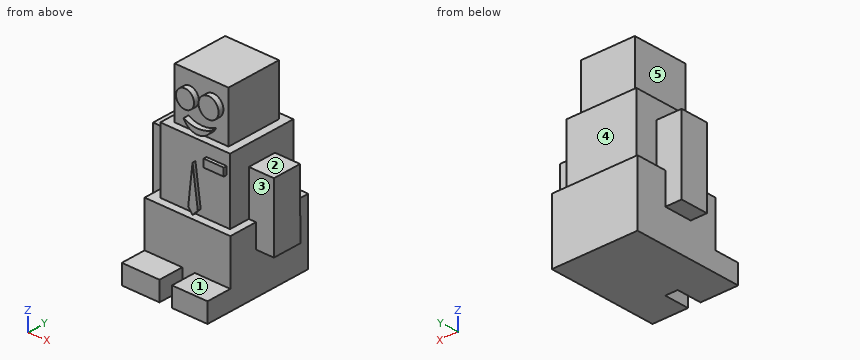
from build123d import *

# Parameters (mm, degrees)
F0_W      = 86.6950079799
F0_H      = 86.6950042546
F1_DEPTH  = 64.9986
F2_W      = 70.5124139786
F2_H      = 70.5124102533
F3_DEPTH  = 64.9986
F4_W      = 54.395288229
F4_H      = 56.1221279204
F5_DEPTH  = 50.8
F6_R      = 9.1186421801
F6_R_2    = 10.1513194638
F6_W      = 20.3841309994
F6_H      = 7.7653825283
F7_DEPTH  = 25.4
F8_W      = 29.1201900691
F8_H      = 44.812363273
F9_DEPTH  = 25.4
F10_W     = 29.5586548746
F10_H     = 23.6200721203
F11_DEPTH = 25.4
F12_W     = 28.1495144591
F12_H     = 46.7537163557
F12_H_2   = 31.3854509233
F13_DEPTH = 25.4
F15_DEPTH = 25.4
F16_W     = 38.1280947477
F16_H     = 19.5383913815
F16_W_2   = 35.9481638297
F17_DEPTH = 25.4
F19_DEPTH = 20
F18_W     = 20.3841309994
F18_H     = 7.7653825283
F20_DEPTH = 15


with BuildPart() as f1:
    # F0 (on Top) → F1 (new body)
    with BuildSketch(Plane.XY):
        with Locations((-0.8532218635, 5.3543392569)):
            Rectangle(F0_W, F0_H)
    extrude(amount=F1_DEPTH)

    # F2 (on face) → F3 (join)
    with BuildSketch(Plane.XY.offset(64.9986)):
        with Locations((0, 4.8926975578)):
            Rectangle(F2_W, F2_H)
    extrude(amount=F3_DEPTH)

    # F4 (on face) → F5 (join)
    with BuildSketch(Plane.XY.offset(129.9972)):
        with Locations((0, 4.8926975578)):
            Rectangle(F4_W, F4_H)
    extrude(amount=F5_DEPTH)

    # F6 (on face) → F7 (join)
    with BuildSketch(Plane.XZ.offset(23.1683664024)):
        with Locations((-11.8907419965, 158.3446115255)):
            Circle(F6_R)
        with Locations((11.8907429278, 159.8006188869)):
            Circle(F6_R_2)
        Polygon((5.5813710205, 70.9840506315), (0.2426664723, 110.2963015437), (0.2426664723, 65.1600137353), align=None)
        Polygon((0.2426664723, 65.1600137353), (0.2426664723, 110.2963015437), (-4.1253603995, 70.9840506315), align=None)
        with Locations((21.5974720195, 114.1789928079)):
            Rectangle(F6_W, F6_H)
    extrude(amount=F7_DEPTH)

    # F8 (on face) → F9 (join)
    with BuildSketch(Plane.YZ.offset(35.2562069893)):
        with Locations((5.0960322842, 87.4047816365)):
            Rectangle(F8_W, F8_H)
    extrude(amount=F9_DEPTH)

    # F10 (on face) → F11 (join)
    with BuildSketch(Plane.YZ.offset(35.2562069893)):
        with Locations((5.3152646869, 53.1885639399)):
            Rectangle(F10_W, F10_H)
    extrude(amount=F11_DEPTH)

    # F12 (on face) → F13 (join)
    with BuildSketch(Plane(origin=(-35.2562069893, 0, 0), x_dir=(0, -1, 0), z_dir=(-1, 0, 0))):
        with Locations((-3.6400225945, 88.3754581779)):
            Rectangle(F12_W, F12_H)
        with Locations((-3.6400225945, 49.3058745384)):
            Rectangle(F12_W, F12_H_2)
    extrude(amount=F13_DEPTH)

    # F14 (on face) → F15 (join)
    with BuildSketch(Plane.XZ.offset(23.1683664024)):
        with BuildLine():
            ThreePointArc((14.7383239205, 141.318809308), (0.6673846717, 137.7586777296), (-13.3936218917, 141.3578391075))
            ThreePointArc((-13.3936218917, 141.3578391075), (0.6597323084, 132.2429981429), (14.7383239205, 141.318809308))
        make_face()
    extrude(amount=F15_DEPTH)

    # F16 (on face) → F17 (join)
    with BuildSketch(Plane.XZ.offset(37.9931628704)):
        with Locations((-25.1366784796, 9.7691956908)):
            Rectangle(F16_W, F16_H)
        with Locations((24.5202002116, 9.7691956908)):
            Rectangle(F16_W_2, F16_H)
    extrude(amount=F17_DEPTH)

    # F19 (cut): faces of the model
    f19_faces = [f1.faces().sort_by_distance(p)[0] for p in [
        (-11.8907419965, -48.5683664024, 158.3446115255),
        (11.8907429278, -48.5683664024, 159.8006188869),
        (0.665272449, -48.5683664024, 136.2362272974),
    ]]
    extrude(f19_faces, amount=-F19_DEPTH, mode=Mode.SUBTRACT)

    # F18 (on face) → F20 (cut)
    with BuildSketch(Plane.XZ.offset(48.5683664024)):
        Polygon((5.5813710205, 70.9840506315), (0.2426664723, 110.2963015437), (-4.1253603995, 70.9840506315), (0.2426664723, 65.1600137353), align=None)
        with Locations((21.5974720195, 114.1789928079)):
            Rectangle(F18_W, F18_H)
    extrude(amount=-F20_DEPTH, mode=Mode.SUBTRACT)


solid = f1.part
Verification items for the finished model (mm, model axes). Face numbers are marked on the shaded views. A direction names the side the tool comes from. Give positions to 0.01 mm unless a question says otherwise; leave off trailing zeros. Loops run counter-clockwise (first coordinate to the right, second up) from the corner with the lowest first, then second, coordinate; pieces in that order, holes last.
1. Cross-section at A-A on y = -45. Record the cut outline in (x, z).
Derived:
outline: (-44.2, 0) - (-6.07, 0) - (-6.07, 19.54) - (-44.2, 19.54) - close; (6.55, 0) - (42.49, 0) - (42.49, 19.54) - (6.55, 19.54) - close
2. Go/stop test with flat-tipped pins: P1, Ø10, axis at y = -48.5, z = 14.5, coming from the -X side; P2, Ø5, axis at y = 21.5, z = 151, coming from the +X side; P3, Ø6, axis at x = 12.5, z = 159.5, coming from the -Y side. Record where each tip stops, or that it passes through.
Derived:
P1: stops at x = -44.2
P2: stops at x = 27.2
P3: stops at y = -28.57
3. Cross-section at D-D on y = 38. Record the cut outline in (x, z).
Derived:
outline: (-44.2, 0) - (42.49, 0) - (42.49, 65) - (35.26, 65) - (35.26, 130) - (-35.26, 130) - (-35.26, 65) - (-44.2, 65) - close
4. Cross-section at C-C on x = -39.5. Record the cut outline in (y, z).
Derived:
outline: (-63.39, 0) - (48.7, 0) - (48.7, 65) - (17.71, 65) - (17.71, 111.75) - (-10.43, 111.75) - (-10.43, 65) - (-37.99, 65) - (-37.99, 19.54) - (-63.39, 19.54) - close
5. Material ranges on probe 1 along Z at (x, y) = (35, -15.5); probe 2 along Z at (x, y) = (10.5, -57.5); probe 3 along X at (y, z) = (36.5, 88), recorded low to high.
Derived:
probe 1: z = 0 to 130
probe 2: z = 0 to 19.54
probe 3: x = -35.26 to 35.26
6. Cross-section at B-B on z = 49. Record the cut outline in (x, y), and give its area (3 significant figures).
Derived:
outline: (-60.66, -10.43) - (-44.2, -10.43) - (-44.2, -37.99) - (42.49, -37.99) - (42.49, -9.46) - (60.66, -9.46) - (60.66, 20.09) - (42.49, 20.09) - (42.49, 48.7) - (-44.2, 48.7) - (-44.2, 17.71) - (-60.66, 17.71) - close
area: 8,520 mm2
7. Tool access check on the marked faces 1, 2, 3, 4 and 5. Record the directions out of +Z, -Z, +X, -X, +Y, -Y that give a thin tool (end or side, any length) a straight path to the whole face; none if there is none.
Derived:
face 1: +Z, +X, -X, -Y
face 2: +Z, +X, +Y, -Y
face 3: +Z, +X, -Y
face 4: +Z, +X, -X, +Y
face 5: +Z, -X, +Y, -Y
